Input: part model. Units: mm. Frame: model coordinates. Coordinates: 2 decimals unless noted, no trailing zeros. Write each loop counter-clockwise with the first axis right and the second up, starting at its lowest first coordinate (ties: lowest second). Pieces come first, ordered by that corner, then holes.
from build123d import *

# Parameters (mm, degrees)
SKETCH_1_W          = 4
SKETCH_1_H          = 7
EXTRUDE_2_DEPTH     = 1
CUT_EXTRUDE_1_DEPTH = 0.2
CUT_EXTRUDE_3_DEPTH = 0.2
SWEEP_1_PROFILE_R   = 0.1
SWEEP_2_PROFILE_R   = 0.1


with BuildPart() as part:
    # 草图1 → 凸台-拉伸2 (new body)
    with BuildSketch(Plane.XY):
        Rectangle(SKETCH_1_W, SKETCH_1_H)
    extrude(amount=EXTRUDE_2_DEPTH)

    # 草图2 → 切除-拉伸1 (cut)
    with BuildSketch(Plane(origin=(0, 0, 0), x_dir=(-1, 0, 0), z_dir=(0, 0, -1))):
        Polygon((1, -3.5), (2, -2.5), (2, -1.5), (0, -3.5), align=None)
        Polygon((-1, -3.5), (2, -0.5), (2, 0.5), (-2, -3.5), align=None)
        Polygon((-2, -2.5), (2, 1.5), (2, 2.5), (-2, -1.5), align=None)
        Polygon((2, 4), (-2, 0), (-2, -0.5), (2, 3.5), align=None)
        Polygon((-2, 1), (0.5, 3.5), (-0.5, 3.5), (-2, 2), align=None)
        Polygon((-2, 3), (-1.5, 3.5), (-2, 3.5), align=None)
    extrude(amount=-CUT_EXTRUDE_1_DEPTH, mode=Mode.SUBTRACT)

    # 草图4 → 切除-拉伸3 (cut)
    with BuildSketch(Plane.XY):
        Polygon((1, -4), (2, -3), (2, -2), (0, -4), align=None)
        Polygon((-1, -4), (2, -1), (2, 0), (-2, -4), align=None)
        Polygon((-2, -3), (2, 1), (2, 2), (-2, -2), align=None)
        Polygon((2, 4), (-2, 0), (-2, -1), (2, 3), align=None)
        Polygon((-2, 1), (1, 4), (0, 4), (-2, 2), align=None)
        Polygon((-2, 3), (-1, 4), (-2, 4), align=None)
    extrude(amount=CUT_EXTRUDE_3_DEPTH, mode=Mode.SUBTRACT)

    # 扫描1: sweep along a path in 草图5
    with BuildLine(Plane.XY.offset(0.5)) as sweep_1_path:
        Line((1.25, -3.5), (1.25, -8.5))
    # 扫描1 profile (on start of the path) → 扫描1 (sweep)
    with BuildSketch(Plane(origin=(1.25, -3.5, 0.5), x_dir=(-1, 0, 0), z_dir=(0, -1, 0))):
        Circle(SWEEP_1_PROFILE_R)
    sweep(path=sweep_1_path.line)

    # 扫描2: sweep along a path in 草图18
    with BuildLine(Plane.XY.offset(0.5)) as sweep_2_path:
        Line((-0.75, -3.5), (-0.75, -8.5))
    # 扫描2 profile (on start of the path) → 扫描2 (sweep)
    with BuildSketch(Plane(origin=(-0.75, -3.5, 0.5), x_dir=(-1, 0, 0), z_dir=(0, -1, 0))):
        Circle(SWEEP_2_PROFILE_R)
    sweep(path=sweep_2_path.line)


solid = part.part
Item 1: Section query A-A, the plane y = -5.25. Return loops of the section in (x, z).
Item 2: Pull-direction query (X, two-part tool) for faces 1 (the face through (-0.8, 1.8, 0)), 2 (the face through (2, 0, 0.6)), 3 (the face through (0, 0, 0.2)); classes: released by +X, released by -X, zero draft, split by the parting line, or undercut.
Item 3: Material intervals for line 1 (Z direction, x = -0.3, y = 2); line 2 (Y direction, x = 1.35, z = 0.4); line 3 (X direction, y = -5.75, z = 0.45), sorted ascending.
The answers:
1. outline: circle Ø0.2 at (-0.75, 0.5); circle Ø0.2 at (1.25, 0.5)
2. face 1: zero draft
2. face 2: released by +X
2. face 3: undercut
3. line 1: z = 0.2 to 1
3. line 2: y = -3.5 to 3.5
3. line 3: x = -0.84 to -0.66, 1.16 to 1.34
